Source: CAD feature listing. Evaluate the final solid. Frame: model axes, mm. Face numbers are marked on the shaded views. A direction names the side the tool comes from. Give positions to 0.01 mm unless a question says otherwise; leave off trailing zeros. Loops run counter-clockwise (first coordinate to the right, second up) from the corner with the lowest first, then second, coordinate; pieces in that order, holes last.
from build123d import *

# Parameters (mm, degrees)
SKETCH_1_R          = 4
EXTRUDE_1_DEPTH     = 5
CUT_EXTRUDE_1_DEPTH = 3.4
SKETCH_3_R          = 2.309401077
CUT_EXTRUDE_2_DEPTH = 3.4
CUT_EXTRUDE_2_DRAFT = -45
CHAMFER_1_SIZE      = 0.2
SKETCH_4_R          = 2.5
EXTRUDE_2_DEPTH     = 8
CHAMFER_2_SIZE      = 0.2


with BuildPart() as part:
    # Эскиз1 → Бобышка-Вытянуть1 (new body)
    with BuildSketch(Plane.XY):
        Circle(SKETCH_1_R)
    extrude(amount=EXTRUDE_1_DEPTH)

    # Эскиз2 → Вырез-Вытянуть1 (cut)
    with BuildSketch(Plane.XY.offset(5)):
        Polygon((2.309401077, 0), (1.154700538, 2), (-1.154700538, 2), (-2.309401077, 0), (-1.154700538, -2), (1.154700538, -2), align=None)
    extrude(amount=-CUT_EXTRUDE_1_DEPTH, mode=Mode.SUBTRACT)


with BuildPart() as cut_extrude_2_tool:
    # Эскиз3 → Вырез-Вытянуть2 (with draft: the straight prism first)
    with BuildSketch(Plane.XY.offset(5)):
        Circle(SKETCH_3_R)
    extrude(amount=-CUT_EXTRUDE_2_DEPTH)
    # Вырез-Вытянуть2: the draft: its side faces are tilted about the plane it starts from
    cut_extrude_2_sides = [cut_extrude_2_tool.faces().sort_by_distance(p)[0] for p in [
        (-2.309401077, 0, 3.3),
    ]]
    draft(cut_extrude_2_sides, Plane.XY.offset(5), CUT_EXTRUDE_2_DRAFT)


with BuildPart() as part_1:
    add(part.part)

    # Вырез-Вытянуть2: cut by cut_extrude_2_tool
    add(cut_extrude_2_tool.part, mode=Mode.SUBTRACT)

    # Фаска1
    chamfer_1_edges = [part_1.edges().sort_by_distance(p)[0] for p in [
        (-4, 0, 5),
    ]]
    chamfer(chamfer_1_edges, length=CHAMFER_1_SIZE)

    # Эскиз4 → Бобышка-Вытянуть2 (add)
    with BuildSketch(Plane(origin=(0, 0, 0), x_dir=(-1, 0, 0), z_dir=(0, 0, -1))):
        Circle(SKETCH_4_R)
    extrude(amount=EXTRUDE_2_DEPTH)

    # Фаска2
    chamfer_2_edges = [part_1.edges().sort_by_distance(p)[0] for p in [
        (2.5, 0, -8),
    ]]
    chamfer(chamfer_2_edges, length=CHAMFER_2_SIZE)


solid = part_1.part
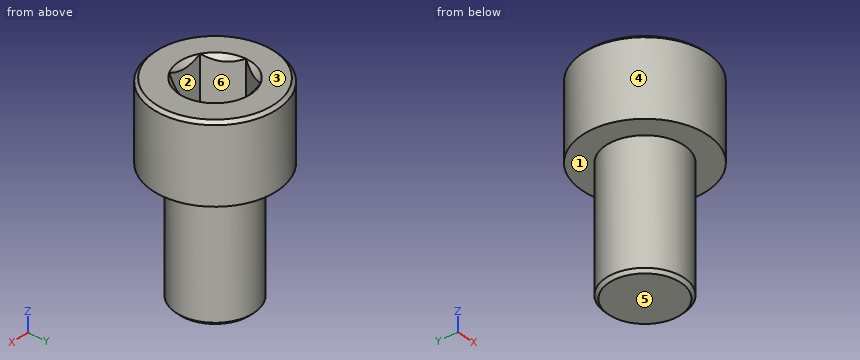
1) Cut plane A-A (z = 3). Return loops of the section in (x, y).
Checks:
outline: circle Ø8 at (0, 0); hole (-2.31, 0) - (-1.15, -2) - (1.15, -2) - (2.31, 0) - (1.15, 2) - (-1.15, 2) - close
2) Pull-direction query (X, two-part tool) for the marked faces 4, 5 and 6; classes: released by +X, released by -X, zero draft, split by the parting line, or undercut.
Checks:
face 4: split by the parting line
face 5: zero draft
face 6: undercut
3) Cut plane C-C (z = -4.75). Return loops of the section in (x, y).
Checks:
outline: circle Ø5 at (0, 0)
4) Contact query for flat-ended pins moving along their axis: P1, Ø1.5, axis at x = 1, z = 0.5, coming from the +Y side; P2, Ø1.5, axis at x = -3, z = -4.5, coming from the -Y side; P3, Ø3, axis at y = 1.5, z = -3.5, coming from the -X side. Output: stop coordinate, or through.
Checks:
P1: stops at y = 3.99
P2: stops at y = -1.09
P3: stops at x = -2.5
5) Cut plane B-B (x = 0). Return loops of the section in (y, z).
Checks:
outline: (-4, 0) - (-2.5, 0) - (-2.5, -7.8) - (-2.3, -8) - (2.3, -8) - (2.5, -7.8) - (2.5, 0) - (4, 0) - (4, 4.8) - (3.8, 5) - (2.31, 5) - (2, 4.69) - (2, 1.6) - (-2, 1.6) - (-2, 4.69) - (-2.31, 5) - (-3.8, 5) - (-4, 4.8) - close
6) Reachability of the marked faces 1, 2 and 3 from +Z, -Z, +X, -X, +Y, -Y: full face, straight path, thin tool, end or side. Return the list, or none.
Checks:
face 1: -Z
face 2: +Z
face 3: +Z, +X, -X, +Y, -Y
7) Ray query, probe 1 along Y at (x, z) = (-1.5, -1.25); probe 2 along Z at (x, y) = (2.75, -1.5); probe 3 along Z at (x, y) = (0.75, -0.75). Return the intervals inside material, ascending.
Checks:
probe 1: y = -2 to 2
probe 2: z = 0 to 5
probe 3: z = -8 to 1.6
